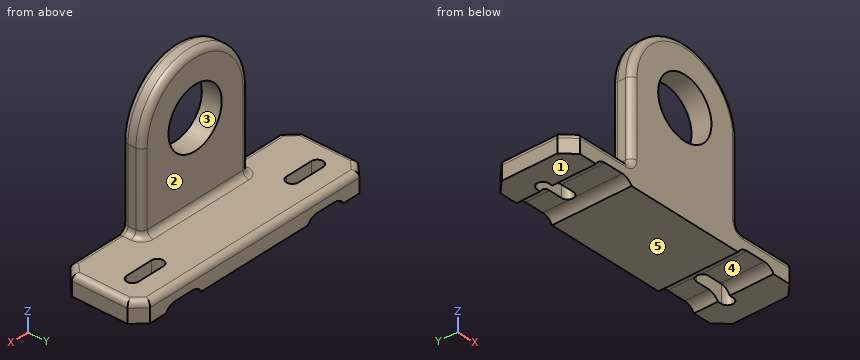
from build123d import *

# Parameters (mm, degrees)
ESQUISSE1_W             = 130
ESQUISSE1_H             = 40
BOSS_EXTRU_1_DEPTH      = 10
ESQUISSE2_R             = 15
BOSS_EXTRU_2_DEPTH      = 10
ENL_V_MAT_EXTRU_1_DEPTH = 98.59610648
ESQUISSE4_W             = 20
ESQUISSE4_H             = 3
ENL_V_MAT_EXTRU_2_DEPTH = 111.566721937
CONG_1_R                = 6
CONG_1_OF_SYM_TRIE2_R   = 6
CHANFREIN1_SIZE         = 6
CONG_2_R                = 3


with BuildPart() as part:
    # Esquisse1 → Boss.-Extru.1 (new body)
    with BuildSketch(Plane.XY):
        Rectangle(ESQUISSE1_W, ESQUISSE1_H)
    extrude(amount=BOSS_EXTRU_1_DEPTH)

    # Esquisse2 → Boss.-Extru.2 (add)
    with BuildSketch(Plane.XZ.offset(20)):
        with BuildLine():
            Line((-30, 0), (-30, 50))
            ThreePointArc((-30, 50), (0, 80), (30, 50))
            Line((30, 50), (30, 0))
            Line((30, 0), (-30, 0))
        make_face()
        with Locations(Location((0, 50, 0), (0, 0, 270))):
            Circle(ESQUISSE2_R, mode=Mode.SUBTRACT)
    extrude(amount=-BOSS_EXTRU_2_DEPTH)

    # Esquisse3 → Enlèv. mat.-Extru.1 (cut, through all)
    with BuildSketch(Plane.XY.offset(10)):
        with BuildLine():
            Line((38, 8), (52, 8))
            ThreePointArc((52, 8), (55, 5), (52, 2))
            Line((52, 2), (38, 2))
            ThreePointArc((38, 2), (35, 5), (38, 8))
        make_face()
    enl_v_mat_extru_1 = extrude(amount=-ENL_V_MAT_EXTRU_1_DEPTH, mode=Mode.SUBTRACT)

    # Symétrie1: Enlèv. mat.-Extru.1 across plane
    add(enl_v_mat_extru_1.mirror(Plane(origin=(0, 0, 0), x_dir=(0, 0, 1), z_dir=(1, 0, 0))), mode=Mode.SUBTRACT)

    # Esquisse4 → Enlèv. mat.-Extru.2 (cut, through all)
    with BuildSketch(Plane.XZ.offset(20)):
        with Locations((40, 1.5)):
            Rectangle(ESQUISSE4_W, ESQUISSE4_H)
    enl_v_mat_extru_2 = extrude(amount=-ENL_V_MAT_EXTRU_2_DEPTH, mode=Mode.SUBTRACT)

    # Congé1
    # the kernel refuses this fillet: 6 mm, written as the material it adds along each edge
    with BuildSketch(Plane(origin=(50, -20, 3), x_dir=(-1, 0, 0), z_dir=(0, 1, 0))) as cong_1_piece_1:
        with BuildLine():
            CenterArc((5.196152423, -6), CONG_1_R, 90, 60)
            Line((0, -3), (-0.103923048, -2.94))
            ThreePointArc((-0.103923048, -2.94), (-0.12, -1.5), (-0.12, 0))
            Line((-0.12, 0), (0, 0.12))
            Line((0, 0.12), (5.196152423, 0.12))
            Line((5.196152423, 0.12), (5.196152423, 0))
        make_face()
    extrude(amount=22)
    with BuildSketch(Plane(origin=(50, -20, 3), x_dir=(-1, 0, 0), z_dir=(0, 1, 0))) as cong_1_piece_2_section:
        with BuildLine():
            CenterArc((5.196152423, -6), CONG_1_R, 90, 60)
            Line((0, -3), (-0.103923048, -2.94))
            ThreePointArc((-0.103923048, -2.94), (-0.12, -1.5), (-0.12, 0))
            Line((-0.12, 0), (0, 0.12))
            Line((0, 0.12), (5.196152423, 0.12))
            Line((5.196152423, 0.12), (5.196152423, 0))
        make_face()
    cong_1_piece_2 = extrude(amount=34.990381057, mode=Mode.PRIVATE)
    cong_1_piece_2 = split(cong_1_piece_2, bisect_by=Plane(origin=(48.702137325, 8, 2.222899734), z_dir=(0, 1, 0)), keep=Keep.TOP, mode=Mode.PRIVATE)
    add(cong_1_piece_2)
    with BuildSketch(Plane(origin=(50, -4.990381057, 3), x_dir=(-1, 0, 0), z_dir=(0, 1, 0))) as cong_1_piece_3_section:
        with BuildLine():
            CenterArc((5.196152423, -6), CONG_1_R, 90, 60)
            Line((0, -3), (-0.103923048, -2.94))
            ThreePointArc((-0.103923048, -2.94), (-0.12, -1.5), (-0.12, 0))
            Line((-0.12, 0), (0, 0.12))
            Line((0, 0.12), (5.196152423, 0.12))
            Line((5.196152423, 0.12), (5.196152423, 0))
        make_face()
    cong_1_piece_3 = extrude(amount=24.990381057, mode=Mode.PRIVATE)
    cong_1_piece_3 = split(cong_1_piece_3, bisect_by=Plane(origin=(48.702137325, 2, 2.222899734), z_dir=(0, -1, 0)), keep=Keep.TOP, mode=Mode.PRIVATE)
    add(cong_1_piece_3)
    with BuildSketch(Plane(origin=(50, 8, 3), x_dir=(-1, 0, 0), z_dir=(0, 1, 0))) as cong_1_piece_4:
        with BuildLine():
            CenterArc((5.196152423, -6), CONG_1_R, 90, 60)
            Line((0, -3), (-0.103923048, -2.94))
            ThreePointArc((-0.103923048, -2.94), (-0.12, -1.5), (-0.12, 0))
            Line((-0.12, 0), (0, 0.12))
            Line((0, 0.12), (5.196152423, 0.12))
            Line((5.196152423, 0.12), (5.196152423, 0))
        make_face()
    extrude(amount=12)
    with BuildSketch(Plane(origin=(30, -20, 3), x_dir=(0, 0, -1), z_dir=(0, 1, 0))) as cong_1_piece_5_section:
        with BuildLine():
            CenterArc((6, -5.196152423), CONG_1_R, 120, 60)
            Line((0, -5.196152423), (-0.12, -5.196152423))
            Line((-0.12, -5.196152423), (-0.12, 0))
            Line((-0.12, 0), (0, 0.12))
            ThreePointArc((0, 0.12), (1.5, 0.12), (2.94, 0.103923048))
            Line((2.94, 0.103923048), (3, 0))
        make_face()
    cong_1_piece_5 = extrude(amount=40, mode=Mode.PRIVATE)
    cong_1_piece_5 = cong_1_piece_5 - Plane(origin=(38, 5, 2.222770997), x_dir=(0, -1, 0), z_dir=(0, 0, 1)) * Cylinder(3, 101, mode=Mode.PRIVATE)
    add(cong_1_piece_5)

    # Symétrie2: Enlèv. mat.-Extru.2 across plane
    add(enl_v_mat_extru_2.mirror(Plane(origin=(0, 0, 0), x_dir=(0, 0, 1), z_dir=(1, 0, 0))), mode=Mode.SUBTRACT)

    # Congé1 of Symétrie2
    # the kernel refuses this fillet: 6 mm, written as the material it adds along each edge
    with BuildSketch(Plane(origin=(-50, -20, 3), x_dir=(1, 0, 0), z_dir=(0, 1, 0))) as cong_1_of_sym_trie2_piece_1:
        with BuildLine():
            CenterArc((5.196152423, 6), CONG_1_OF_SYM_TRIE2_R, 210, 60)
            Line((0, 3), (-0.103923048, 2.94))
            ThreePointArc((-0.103923048, 2.94), (-0.12, 1.5), (-0.12, 0))
            Line((-0.12, 0), (0, -0.12))
            Line((0, -0.12), (5.196152423, -0.12))
            Line((5.196152423, -0.12), (5.196152423, 0))
        make_face()
    extrude(amount=22)
    with BuildSketch(Plane(origin=(-50, -20, 3), x_dir=(1, 0, 0), z_dir=(0, 1, 0))) as cong_1_of_sym_trie2_piece_2_section:
        with BuildLine():
            CenterArc((5.196152423, 6), CONG_1_OF_SYM_TRIE2_R, 210, 60)
            Line((0, 3), (-0.103923048, 2.94))
            ThreePointArc((-0.103923048, 2.94), (-0.12, 1.5), (-0.12, 0))
            Line((-0.12, 0), (0, -0.12))
            Line((0, -0.12), (5.196152423, -0.12))
            Line((5.196152423, -0.12), (5.196152423, 0))
        make_face()
    cong_1_of_sym_trie2_piece_2 = extrude(amount=34.990381057, mode=Mode.PRIVATE)
    cong_1_of_sym_trie2_piece_2 = split(cong_1_of_sym_trie2_piece_2, bisect_by=Plane(origin=(-48.702137325, 8, 2.222899734), z_dir=(0, 1, 0)), keep=Keep.TOP, mode=Mode.PRIVATE)
    add(cong_1_of_sym_trie2_piece_2)
    with BuildSketch(Plane(origin=(-50, -4.990381057, 3), x_dir=(1, 0, 0), z_dir=(0, 1, 0))) as cong_1_of_sym_trie2_piece_3_section:
        with BuildLine():
            CenterArc((5.196152423, 6), CONG_1_OF_SYM_TRIE2_R, 210, 60)
            Line((0, 3), (-0.103923048, 2.94))
            ThreePointArc((-0.103923048, 2.94), (-0.12, 1.5), (-0.12, 0))
            Line((-0.12, 0), (0, -0.12))
            Line((0, -0.12), (5.196152423, -0.12))
            Line((5.196152423, -0.12), (5.196152423, 0))
        make_face()
    cong_1_of_sym_trie2_piece_3 = extrude(amount=24.990381057, mode=Mode.PRIVATE)
    cong_1_of_sym_trie2_piece_3 = split(cong_1_of_sym_trie2_piece_3, bisect_by=Plane(origin=(-48.702137325, 2, 2.222899734), z_dir=(0, -1, 0)), keep=Keep.TOP, mode=Mode.PRIVATE)
    add(cong_1_of_sym_trie2_piece_3)
    with BuildSketch(Plane(origin=(-50, 8, 3), x_dir=(1, 0, 0), z_dir=(0, 1, 0))) as cong_1_of_sym_trie2_piece_4:
        with BuildLine():
            CenterArc((5.196152423, 6), CONG_1_OF_SYM_TRIE2_R, 210, 60)
            Line((0, 3), (-0.103923048, 2.94))
            ThreePointArc((-0.103923048, 2.94), (-0.12, 1.5), (-0.12, 0))
            Line((-0.12, 0), (0, -0.12))
            Line((0, -0.12), (5.196152423, -0.12))
            Line((5.196152423, -0.12), (5.196152423, 0))
        make_face()
    extrude(amount=12)
    with BuildSketch(Plane(origin=(-30, -20, 3), x_dir=(0, 0, -1), z_dir=(0, 1, 0))) as cong_1_of_sym_trie2_piece_5_section:
        with BuildLine():
            CenterArc((6, 5.196152423), CONG_1_OF_SYM_TRIE2_R, 180, 60)
            Line((0, 5.196152423), (-0.12, 5.196152423))
            Line((-0.12, 5.196152423), (-0.12, 0))
            Line((-0.12, 0), (0, -0.12))
            ThreePointArc((0, -0.12), (1.5, -0.12), (2.94, -0.103923048))
            Line((2.94, -0.103923048), (3, 0))
        make_face()
    cong_1_of_sym_trie2_piece_5 = extrude(amount=40, mode=Mode.PRIVATE)
    cong_1_of_sym_trie2_piece_5 = cong_1_of_sym_trie2_piece_5 - Plane(origin=(-38, 5, 2.222770997), x_dir=(0, -1, 0), z_dir=(0, 0, 1)) * Cylinder(3, 101, mode=Mode.PRIVATE)
    add(cong_1_of_sym_trie2_piece_5)

    # Chanfrein1
    chanfrein1_edges = [part.edges().sort_by_distance(p)[0] for p in [
        (-65, -20, 5),
        (65, -20, 5),
        (65, 20, 5),
        (-65, 20, 5),
    ]]
    chamfer(chanfrein1_edges, length=CHANFREIN1_SIZE)

    # Congé2
    cong_2_edges = [part.edges().sort_by_distance(p)[0] for p in [
        (-65, 0, 10),
        (0, 20, 10),
        (-44.5, -20, 10),
        (65, 0, 10),
        (-62, -17, 10),
        (62, -17, 10),
        (62, 17, 10),
        (-62, 17, 10),
        (44.5, -20, 10),
        (-30, -10, 30),
        (30, -10, 30),
        (-30, -20, 30),
        (30, -20, 30),
        (0, -20, 80),
        (-30, -15, 10),
        (0, -10, 80),
        (30, -15, 10),
        (0, -10, 10),
    ]]
    fillet(cong_2_edges, radius=CONG_2_R)


solid = part.part
The model under review builds one solid part; all positions refer to its coordinate system, in mm. Face numbers are marked on the shaded views. A direction names the side the tool comes from. Give positions to 0.01 mm unless a question says otherwise; leave off trailing zeros. Order: outer loops, then holes, each group sorted by start corner. A loop starts at its lowest first (then second) coordinate and runs counter-clockwise, first axis right, second up. Notation, with made-up numbers: M 29.5,10.25 L 65.5,10.25 A13 ccw 65.5,27.25 Z; hole C -27,-29 d8. An arc over 180 degrees is marked long. Use one line per item in the form item = value. Start each with the question number.
Item 1: The part is to be moulded in two halves that separate along Z. For the marked faces 1, 2 and 3, say which applies: pulls with the +Z half, pulls with the -Z half, needs draft (parallel to the pull), parting line crosses it, or undercut.
Item 2: We need section C-C on x = 0. Give the boundary of the cut face in (y, z).
Item 3: We need section A-A on x = 42. Give the boundary of the cut face in (y, z), plus the area to 3 significant figures.
Item 4: Insertion check: pin 1 Ø10 at (x, z) = (29, 23.5) entering from -Y; pin 2 Ø12 at (y, z) = (-5.5, 27.5) entering from -X; pin 3 Ø10 at (y, z) = (-13.5, 56.5) entering from +X; pin 4 Ø6 at (x, z) = (-39.5, 12) entering from +Y. Each pin has a flat end and moves straight along its axis. Give the tip position at first contact, or say it passes through.
Item 5: We need section B-B on z = 22. Give the boundary of the cut face in (x, y).
Item 6: For the marked faces 4 and 5, list the 3-axis set-ups (+Z, -Z, +X, -X, +Y, -Y) from which the entire face can be reached by the end or side of a thin tool; tool diameter is ignored.
Item 7: To check wall thickness, follow line 1 along X through (y, z) = (-14.75, 50); line 2 along X through (y, z) = (6, 4.5); line 3 along Z through (x, y) = (29, 1). State the ranges of each line that lie inside material, in increasing order. Write a range as from..to.
Completed:
q1.face_1 = pulls with the -Z half
q1.face_2 = needs draft
q1.face_3 = undercut
q2.outline = M -20,0 L 20,0 L 20,7 A3 ccw 17,10 L -7,10 A3 cw -10,13 L -10,35 L -20,35 Z; M -20,65 L -10,65 L -10,77 A3 ccw -13,80 L -17,80 A3 ccw -20,77 Z
q3.outline = M -20,3 L 2,3 L 2,10 L -17,10 A3 ccw -20,7 Z; M 8,3 L 20,3 L 20,7 A3 ccw 17,10 L 8,10 Z
q3.area = 234 mm²
q4.pin_1 = -20
q4.pin_2 = -29.6
q4.pin_3 = 29.96
q4.pin_4 = 19.24
q5.outline = M -30,-17 A3 ccw -27,-20 L 27,-20 A3 ccw 30,-17 L 30,-13 A3 ccw 27,-10 L -27,-10 A3 ccw -30,-13 Z
q6.face_4 = -Z, +Y, -Y
q6.face_5 = -Z, +X, -X, +Y, -Y
q7.line_1 = -30..-15, 15..30
q7.line_2 = -65..-54.83, -35.17..35.17, 54.83..65
q7.line_3 = 0..10
